Here's how the part is built. I have some questions about the finished solid (model axes, mm). A direction names the side the tool comes from. Coordinates: 2 decimals unless noted, no trailing zeros. Write each loop counter-clockwise with the first axis right and the second up, starting at its lowest first coordinate (ties: lowest second). Pieces come first, ordered by that corner, then holes.
Item 1: I want a section at A-A (z = -68). Please give me the cut outline in (x, y), and give its area (3 significant figures).
Item 2: I want a section at B-B (x = 13). Please give me the cut outline in (y, z), and give its area (3 significant figures).
Item 3: If we mould it in two halves opening along Z, with no side actions, what happens to faces 4 (the face through (0, -120, 58.496)), 5 (the face through (0, -99.989, 29)), 6 (the face through (0, 55.998, -134))? For each: pulls with the +Z half, pulls with the -Z half, needs draft (parallel to the pull), parting line crosses it, or undercut.
Item 4: Please list where these lines run through material, in increasing order: line 1 (Z direction, x = -19.5, y = -94.5); line 2 (Y direction, x = 18.5, z = -51); line 3 (Y direction, x = 6.5, z = -93.5).
Item 5: I want a section at C-C (y = -114). Please give me the cut outline in (x, z), and give its area (3 significant figures).
Item 6: I'm going to push flat-ended pins straight in: P1, Ø23, axis at x = 8.5, z = -78.5, coming from the +Y side; P2, Ø14, axis at x = -1, z = -29, coming from the -Y side; P3, Ø5.5, axis at x = 8, z = 51, coming from the +Y side; P4, Ø10, axis at y = -83, z = -36, coming from the +X side. Where does each tip first touch, or does it pass through?
Item 7: I want a section at D-D (z = -32). Please give me the cut outline in (x, y), and give its area (3 significant figures).
Item 8: For faces 1 (the face through (0, -92.989, 53)), 2 (the face through (0, 0.021, -83)), 3 (the face through (0, -139.989, -7)), which set-ups out of +Z, -Z, +X, -X, +Y, -Y let a thin tool reach every point of the face, with its end or its side?
Autodesk Inventor part; units mm, degrees
ref_plane "YZ Plane" through (0, 0, 0) normal (1, 0, 0) x (0, 1, 0)
ref_plane "XZ Plane" through (0, 0, 0) normal (0, 1, 0) x (-1, 0, 0)
ref_plane "XY Plane" through (0, 0, 0) normal (0, 0, 1) x (1, 0, 0)
sketch "Sketch3" plane through (0, 0, 0) normal (1, 0, 0) x (0, 1, 0)
  line L0 (0, 0) -> (48.9982, 0)
  line L1 (48.9982, -15.0415) -> (48.9982, -124.2618)
  line L2 (48.9982, -139.3032) -> (0.0211, -139.3032)
  line L3 (0.0211, -124.2618) -> (0.0211, -41.5471)
  line L4 (0, 0) -> (-99.9892, 13.7012)
  line L5 (-99.9892, -27.843) -> (0.0211, -41.5471)
  line L6 (48.9982, -139.3032) -> (55.9982, -139.3032)
  line L7 (55.9982, -139.3032) -> (55.9982, -128.3032)
  line L8 (55.9982, -128.3032) -> (48.9982, -124.2618)
  line L9 (48.9982, 0) -> (55.9982, 0)
  line L10 (55.9982, 0) -> (55.9982, -11)
  line L11 (55.9982, -11) -> (48.9982, -15.0415)
  line L12 (0.0211, -139.3032) -> (-6.9789, -139.3032)
  line L13 (-6.9789, -139.3032) -> (-6.9789, -128.3032)
  line L14 (-6.9789, -128.3032) -> (0.0211, -124.2618)
  line L15 (-148.6902, -63.3226) -> (-148.65, -63.3226)
  line L16 (-99.9892, -27.843) -> (-99.9892, -56.4562)
  line L17 (-99.9789, -71.5036) -> (-139.9913, -71.5036)
  line L18 (-139.9892, -56.4622) -> (-139.9892, 43.4549)
  line L19 (-139.9892, 58.4964) -> (-99.9892, 58.4964)
  line L20 (-99.9892, 43.4549) -> (-99.9892, 13.7012)
  line L21 (-99.9789, -71.5036) -> (-92.9789, -71.5036)
  line L22 (-92.9789, -71.5036) -> (-92.9789, -60.5036)
  line L23 (-92.9789, -60.5036) -> (-99.9892, -56.4562)
  line L24 (-139.9913, -71.5036) -> (-146.9913, -71.5036)
  line L25 (-146.9913, -71.5036) -> (-146.9913, -60.5036)
  line L26 (-146.9913, -60.5036) -> (-139.9892, -56.4622)
  line L27 (-139.9892, 58.4964) -> (-146.9892, 58.4964)
  line L28 (-146.9892, 58.4964) -> (-146.9892, 47.4964)
  line L29 (-146.9892, 47.4964) -> (-139.9892, 43.4549)
  line L30 (-99.9892, 58.4964) -> (-92.9892, 58.4964)
  line L31 (-92.9892, 58.4964) -> (-92.9892, 47.4964)
  line L32 (-92.9892, 47.4964) -> (-99.9892, 43.4549)
  dimension "d11" = 120
  dimension "d12" = 7
  dimension "d13" = 11
  dimension "d16" = 130
  dimension "d17" = 40
  dimension "d18" = 7
  dimension "d19" = 11
  dimension "d20" = 120
  dimension "d21" = 120
extrude "Extrusion1" add sketch "Sketch3" along normal mid plane 46
sketch "Sketch4" plane through (23, 0.0211, -41.5471) normal (0, -0.1358, -0.9907) x (-1, 0, 0)
  line L0 (0, -5.6613) -> (0, -106.5849)
  line L1 (4.6881, -26.5876) -> (4.6881, -87.9351)
  line L2 (4.6881, -87.9351) -> (0, -92.5468)
  line L3 (-2.0913, -87.9351) -> (56.7354, -87.9351) construction
  line L4 (4.6881, -26.5876) -> (0, 0)
  line L5 (46, 0) -> (0, 0)
  line L6 (-9.1248, -26.5258) -> (54.948, -26.5258) construction
  line L7 (46, 0) -> (46, -100.9449)
  line L8 (46, 0) -> (41.3228, -26.5258)
  line L9 (41.3228, -26.5258) -> (41.3228, -87.9351)
  line L10 (41.3228, -87.9351) -> (46, -92.5468)
  line L11 (46, -106.5849) -> (46, -5.6613)
  point P0 (23, -5.6613)
  dimension "d25" = 80
  dimension "d26" = 80
sketch "Sketch5" plane through (23, 0.0211, -41.5471) normal (0, -0.1358, -0.9907) x (-1, 0, 0)
  point P0 (23, -5.6613)
properties part number "Big Housing"
Answer:
1. outline: (-23, -146.99) - (23, -146.99) - (23, -92.98) - (-23, -92.98) - close; (-23, 0.02) - (23, 0.02) - (23, 49) - (-23, 49) - close
1. area: 4,740 mm2
2. outline: (-146.99, -71.5) - (-92.98, -71.5) - (-92.98, -60.5) - (-99.99, -56.46) - (-99.99, -27.84) - (0.02, -41.55) - (0.02, -124.26) - (-6.98, -128.3) - (-6.98, -139.3) - (56, -139.3) - (56, -128.3) - (49, -124.26) - (49, -15.04) - (56, -11) - (56, 0) - (0, 0) - (-99.99, 13.7) - (-99.99, 43.45) - (-92.99, 47.5) - (-92.99, 58.5) - (-146.99, 58.5) - (-146.99, 47.5) - (-139.99, 43.45) - (-139.99, -56.46) - (-146.99, -60.5) - close
2. area: 16,800 mm2
3. face 4: pulls with the +Z half
3. face 5: undercut
3. face 6: needs draft
4. line 1: z = -71.5 to -59.63, -28.6 to 12.95, 46.62 to 58.5
4. line 2: y = -139.99 to -99.99, 0.02 to 49
4. line 3: y = 0.02 to 49
5. outline: (-23, -71.5) - (23, -71.5) - (23, 58.5) - (-23, 58.5) - close
5. area: 5,980 mm2
6. P1: stops at y = 49
6. P2: stops at y = -139.99
6. P3: stops at y = -92.99
6. P4: passes through
7. outline: (-23, -139.99) - (23, -139.99) - (23, -99.99) - (-23, -99.99) - close; (-23, -69.65) - (23, -69.65) - (23, 49) - (-23, 49) - close
7. area: 7,300 mm2
8. face 1: +Z, +X, -X, +Y
8. face 2: +X, -X
8. face 3: +X, -X, -Y
